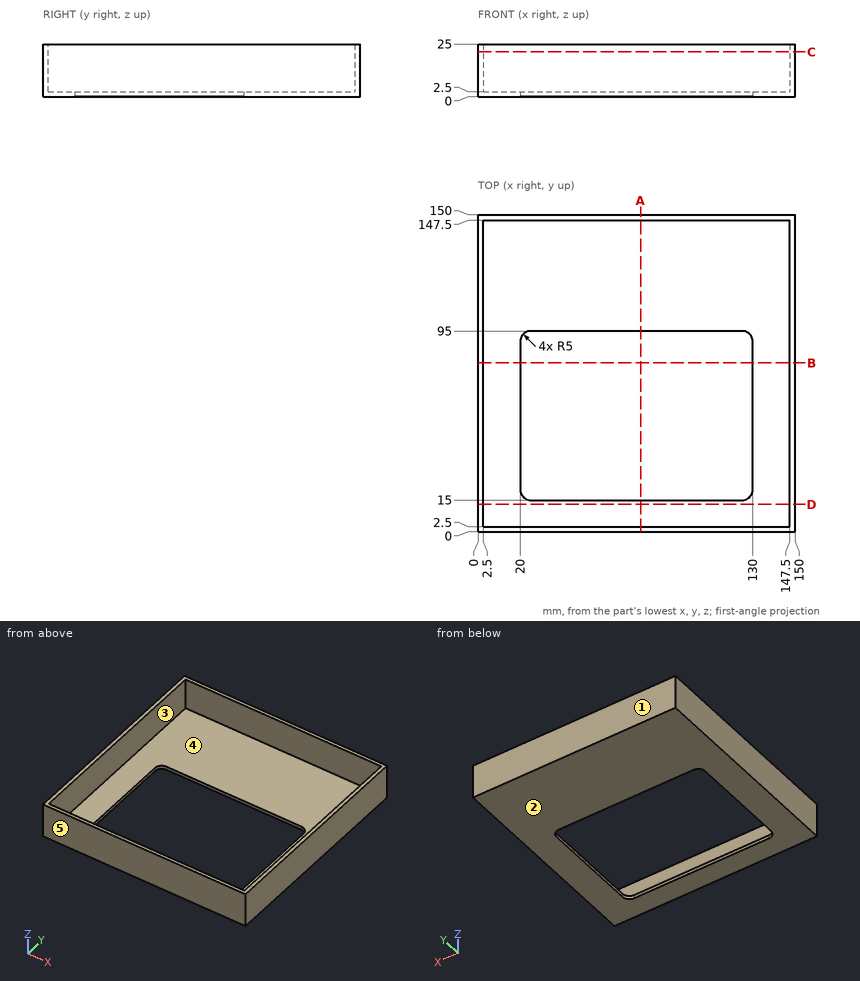
Part print with two shaded views. Sizes in mm from the minimum x, y, z corner. A direction names the side the tool comes from. Give positions to 0.01 mm unless a question says otherwise; leave off trailing zeros. Loops run counter-clockwise (first coordinate to the right, second up) from the corner with the lowest first, then second, coordinate; pieces in that order, holes last. Notation, with made-up numbers: (34, 24) -> (59, 24) arc R22 cw to (59, 50) -> close; hole circle Ø11 at (48, 52.5). An arc over 180 degrees is marked (long way). One line per question, with ' | ' between items.
Q1. Tool access for the marked faces 4 and 5: list every direction of +Z, -Z, +X, -X, +Y, -Y with a clear straight run to the whole face (end or side of a thin tool).
Filled sheet:
face 4: +Z | face 5: +Z, -Z, +X, -X, -Y
Q2. Pull direction Y, two halves, no side cores. Call the marked faces 1, 2 and 3: pulls with the +Y half, pulls with the -Y half, needs draft (parallel to the pull), parting line crosses it, or undercut.
Filled sheet:
face 1: pulls with the +Y half | face 2: needs draft | face 3: undercut
Q3. Cut at C-C, the plane z = 21.25. Write the cut outline in (x, y).
Filled sheet:
outline: (0, 0) -> (150, 0) -> (150, 150) -> (0, 150) -> close; hole (2.5, 2.5) -> (147.5, 2.5) -> (147.5, 147.5) -> (2.5, 147.5) -> close
Q4. Drill centre lines: line 1 along X through (y, z) = (101.5, 19.25); line 2 along Z through (x, y) = (139.5, 45). Where is each one in solid material? Low to high. Write a range as [from, to].
Filled sheet:
line 1: x = [0, 2.5], [147.5, 150] | line 2: z = [0, 2.5]
Q5. Drop flat-ended pins along their axis: pin 1 (8 mm diameter, centred on x = 60, y = 120, fed in from +Z); pin 2 (5 mm diameter, centred on x = 125.5, y = 26.5, fed in from -Z). Give the stop position or say it passes through.
Filled sheet:
pin 1: stops at z = 2.5 | pin 2: passes through
Q6. Cut at B-B, the plane y = 80. Write the cut outline in (x, z), plus the area to 4 significant figures.
Filled sheet:
outline: (0, 0) -> (20, 0) -> (20, 2.5) -> (2.5, 2.5) -> (2.5, 25) -> (0, 25) -> close; (130, 0) -> (150, 0) -> (150, 25) -> (147.5, 25) -> (147.5, 2.5) -> (130, 2.5) -> close | area: 212.5 mm²
Q7. Cut at A-A, the plane x = 77. Write the cut outline in (y, z).
Filled sheet:
outline: (0, 0) -> (15, 0) -> (15, 2.5) -> (2.5, 2.5) -> (2.5, 25) -> (0, 25) -> close; (95, 0) -> (150, 0) -> (150, 25) -> (147.5, 25) -> (147.5, 2.5) -> (95, 2.5) -> close
Q8. Cut at D-D, the plane y = 13. Write the cut outline in (x, z).
Filled sheet:
outline: (0, 0) -> (150, 0) -> (150, 25) -> (147.5, 25) -> (147.5, 2.5) -> (2.5, 2.5) -> (2.5, 25) -> (0, 25) -> close
